Here's the drawing with two shaded views (mm, measured from the low corner). I have some questions. Give positions to 0.01 mm unless a question says otherwise; leave off trailing zeros. Write each loop counter-clockwise with the first axis right and the second up, starting at its lowest first coordinate (ties: lowest second). Pieces come first, ordered by that corner, then holes. Notation, with made-up numbers: M 40.25,20.5 L 68.25,20.5 A8 ccw 68.25,24.5 Z; hole C -11.5,-37 d6. An arc over 180 degrees is marked long. Use one line per item in the form item = value. Start each with the question number.
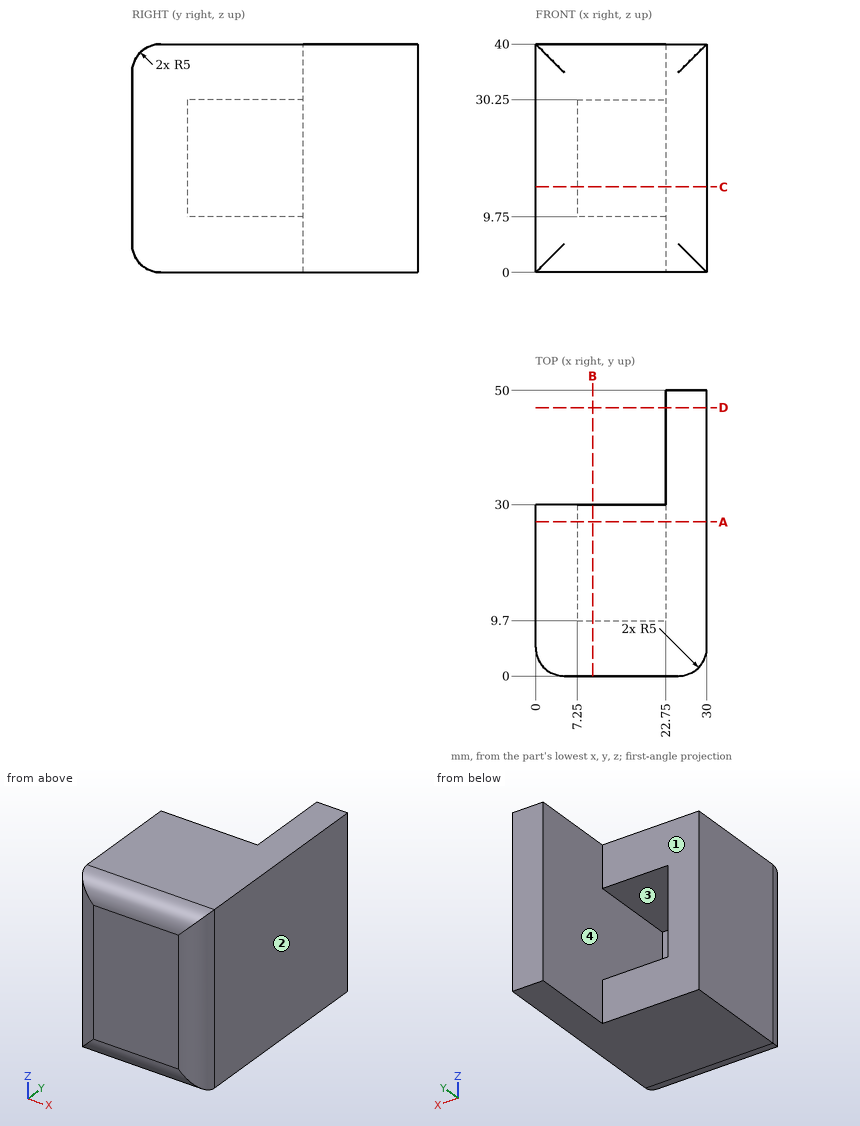
1) Suppose I cut it at C-C, the plane z = 15. List the corners of the cut face in (x, y) for me, and give its area (3 significant figures).
2) Suppose I cut it at D-D, the plane y = 47. List the corners of the cut face in (x, z) for me.
3) Thinking about a two-plate mould opening in X: for the marked faces 1, 2, 3 and 4, which applies, released by +X, released by -X, zero draft, split by the parting line, or undercut?
4) Please list where these lines run through material, in increasing order: line 1 (X direction, y = 13, z = 16); line 2 (Z direction, x = 11.5, y = 26.5); line 3 (X direction, y = 44, z = 25).
5) Will these pins go through, and if not, where does the flat tip stop? P1, Ø2, axis at x = 15.5, z = 16.5, coming from the +Y side; P2, Ø8, axis at x = 10, z = 33, coming from the +Y side.
6) Suppose I cut it at B-B, the plane x = 10. List the corners of the cut face in (y, z) for me, and give its area (3 significant figures).
7) Suppose I cut it at A-A, the plane y = 27. List the corners of the cut face in (x, z) for me, and give its area (3 significant figures).
Checks:
q1.outline = M 0,5 A5 ccw 5,0 L 25,0 A5 ccw 30,5 L 30,50 L 22.75,50 L 22.75,9.7 L 7.25,9.7 L 7.25,30 L 0,30 Z
q1.area = 720 mm^2
q2.outline = M 22.75,0 L 30,0 L 30,40 L 22.75,40 Z
q3.face_1 = zero draft
q3.face_2 = released by +X
q3.face_3 = undercut
q3.face_4 = undercut
q4.line_1 = 0 to 7.25, 22.75 to 30
q4.line_2 = 0 to 9.75, 30.25 to 40
q4.line_3 = 22.75 to 30
q5.P1 = 9.7
q5.P2 = 30
q6.outline = M 0,5 A5 ccw 5,0 L 30,0 L 30,9.75 L 9.7,9.75 L 9.7,30.25 L 30,30.25 L 30,40 L 5,40 A5 ccw 0,35 Z
q6.area = 773 mm^2
q7.outline = M 0,0 L 30,0 L 30,40 L 0,40 Z; hole M 7.25,9.75 L 22.75,9.75 L 22.75,30.25 L 7.25,30.25 Z
q7.area = 882 mm^2
